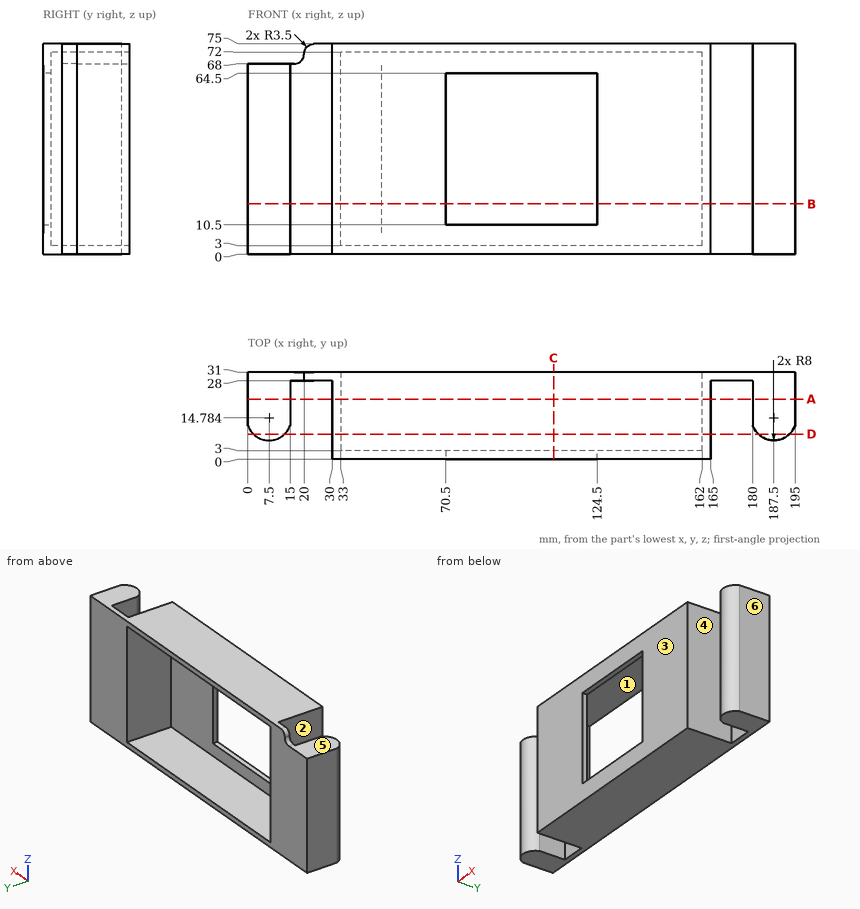
Study the drawing (mm; zero at the part's minimum x, y, z) and answer. A direction names the side the tool comes from. Give positions to 0.01 mm unless a question says otherwise; leave off trailing zeros. Order: outer loops, then holes, each group sorted by start corner. A loop starts at its lowest first (then second) coordinate and runs counter-clockwise, first axis right, second up. Notation, with made-up numbers: (-17, -2) - (2, -2) arc R27 cw to (2, 20) - close; hole circle Ø8 at (-38.5, 17). An arc over 180 degrees is marked (long way). Use one line per item in the form item = value. Start each with the question number.
(1) A cutting plane is placed at C-C, the plane x = 109. Write down the section's boundary in (y, z).
(2) A cutting plane is placed at D-D, the plane y = 9. Write down the section's boundary in (x, z), then the cut area to 3 significant figures.
(3) A cutting plane is placed at A-A, the plane y = 21.5. Write down the section's boundary in (x, z).
(4) For the marked faces 1, 2 and 3, determine the directions among +Z, -Z, +X, -X, +Y, -Y from which every point of the face is accessible in a straight line to the end or side of a thin tool.
(5) Consider line 1 (X direction, y = 27.5, z = 10); line 2 (X direction, y = 13, z = 70); line 3 (X direction, y = 5, z = 4). Determine where each line is inside the solid, lowest interval first. Write a range as from..to.
(6) A cutting plane is placed at B-B, the plane z = 18. Write down the section's boundary in (x, y), then the cut area to 3 significant figures.
(7) Flat-ended cylindrical pins translate along their axes: pin 1 Ø1.5 at (x, z) = (21.5, 43) entering from -Y; pin 2 Ø8.5 at (x, y) = (12, 21) entering from +Z; pin 3 Ø0.9 at (y, z) = (1, 33) entering from +X. Find the tip coordinate at first contact, or state that the pin passes through.
(8) The mould has two halves that part along X. Classify the marked faces 4, 5 and 6: released by +X, released by -X, zero draft, split by the parting line, or undercut.
Ans:
q1.outline = (0, 0) - (31, 0) - (31, 3) - (3, 3) - (3, 10.5) - (0, 10.5) - close; (0, 64.5) - (3, 64.5) - (3, 72) - (31, 72) - (31, 75) - (0, 75) - close
q2.outline = (1.97, 0) - (13.03, 0) - (13.03, 68) - (1.97, 68) - close; (30, 0) - (165, 0) - (165, 75) - (30, 75) - close; (181.97, 0) - (193.03, 0) - (193.03, 75) - (181.97, 75) - close; hole (33, 3) - (162, 3) - (162, 72) - (33, 72) - close
q2.area = 2,800 mm^2
q3.outline = (0, 0) - (15, 0) - (15, 68) - (0, 68) - close; (30, 0) - (165, 0) - (165, 75) - (30, 75) - close; (180, 0) - (195, 0) - (195, 75) - (180, 75) - close; hole (33, 3) - (162, 3) - (162, 72) - (33, 72) - close
q4.face_1 = +Y
q4.face_2 = +Z, -Z, -Y
q4.face_3 = +Z, -Z, +X, -X, -Y
q5.line_1 = 0..15, 30..33, 162..165, 180..195
q5.line_2 = 30..33, 162..165, 180..195
q5.line_3 = 30..33, 162..165
q6.outline = (0, 12) arc R8 ccw to (15, 12) - (15, 28) - (30, 28) - (30, 0) - (70.5, 0) - (70.5, 3) - (33, 3) - (33, 31) - (0, 31) - close; (124.5, 0) - (165, 0) - (165, 28) - (180, 28) - (180, 12) arc R8 ccw to (195, 12) - (195, 31) - (162, 31) - (162, 3) - (124.5, 3) - close
q6.area = 1,180 mm^2
q7.pin_1 = 28
q7.pin_2 = 68
q7.pin_3 = 165
q8.face_4 = undercut
q8.face_5 = zero draft
q8.face_6 = released by +X
